from build123d import *

# Parameters (mm, degrees)
BOSS_EXTRUDE1_DEPTH      = 1.5875
BOSS_EXTRUDE1_DEPTH_BACK = 1.5875
SKETCH3_W                = 0.25
SKETCH3_H                = 13.334960838
SKETCH3_H_2              = 13.334960839
CUT_EXTRUDE1_DEPTH       = 103.531394128
SKETCH4_W                = 0.25
SKETCH4_H                = 6.667480419
SKETCH4_H_2              = 13.334960838
BOSS_EXTRUDE2_DEPTH      = 3.175


with BuildPart() as part:
    # Sketch2 → Boss-Extrude1 (new, two sides: drawn at the far end of the back side and taken through both)
    with BuildSketch(Plane(origin=(0, -26.564964534, 0), x_dir=(1, 0, 0), z_dir=(0, 1, 0)).offset(-BOSS_EXTRUDE1_DEPTH_BACK)):
        Polygon((-40, -26.352441257), (-40, -39.687402095), (-43.675, -39.687402095), (-43.675, -53.022362934), (-40, -53.022362934), (-40, -66.357323772), (-43.675, -66.357323772), (-43.675, -79.69228461), (-40, -79.69228461), (-40, -86.359765029), (-33.083333333, -86.359765029), (-33.083333333, -92.709765029), (-20.25, -92.709765029), (-20.25, -86.359765029), (-6.416666667, -86.359765029), (-6.416666667, -92.709765029), (6.416666667, -92.709765029), (6.416666667, -86.359765029), (20.25, -86.359765029), (20.25, -92.709765029), (33.083333333, -92.709765029), (33.083333333, -86.359765029), (40, -86.359765029), (40, -79.69228461), (43.675, -79.69228461), (43.675, -66.357323772), (40, -66.357323772), (40, -53.022362934), (43.675, -53.022362934), (43.675, -39.687402095), (40, -39.687402095), (40, -26.352441257), (43.675, -26.352441257), (43.675, -13.017480419), (40, -13.017480419), (40, -6.35), (33.083333333, -6.35), (33.083333333, 0), (20.25, 0), (20.25, -6.35), (6.416666667, -6.35), (6.416666667, 0), (-6.416666667, 0), (-6.416666667, -6.35), (-20.25, -6.35), (-20.25, 0), (-33.083333333, 0), (-33.083333333, -6.35), (-40, -6.35), (-40, -13.017480419), (-43.675, -13.017480419), (-43.675, -26.352441257), align=None)
    extrude(amount=BOSS_EXTRUDE1_DEPTH + BOSS_EXTRUDE1_DEPTH_BACK)

    # Sketch3 → Cut-Extrude1 (cut, through all)
    with BuildSketch(Plane(origin=(0, -24.977464534, 0), x_dir=(1, 0, 0), z_dir=(0, 1, 0))):
        with Locations((-43.55, -19.684960838)):
            Rectangle(SKETCH3_W, SKETCH3_H)
        with Locations((-43.55, -46.354882515)):
            Rectangle(SKETCH3_W, SKETCH3_H_2)
        with Locations((-43.55, -73.024804191)):
            Rectangle(SKETCH3_W, SKETCH3_H)
        with Locations((43.55, -19.684960838)):
            Rectangle(SKETCH3_W, SKETCH3_H)
        with Locations((43.55, -46.354882515)):
            Rectangle(SKETCH3_W, SKETCH3_H_2)
        with Locations((43.55, -73.024804191)):
            Rectangle(SKETCH3_W, SKETCH3_H)
    extrude(amount=-CUT_EXTRUDE1_DEPTH, mode=Mode.SUBTRACT)

    # Sketch4 → Boss-Extrude2 (add)
    with BuildSketch(Plane(origin=(0, -24.977464534, 0), x_dir=(1, 0, 0), z_dir=(0, 1, 0))):
        with Locations((-40.125, -9.683740209)):
            Rectangle(SKETCH4_W, SKETCH4_H)
        with Locations((-40.125, -33.019921676)):
            Rectangle(SKETCH4_W, SKETCH4_H_2)
        with Locations((-40.125, -59.689843353)):
            Rectangle(SKETCH4_W, SKETCH4_H_2)
        with Locations((-40.125, -83.02602482)):
            Rectangle(SKETCH4_W, SKETCH4_H)
        with Locations((40.125, -83.02602482)):
            Rectangle(SKETCH4_W, SKETCH4_H)
        with Locations((40.125, -59.689843353)):
            Rectangle(SKETCH4_W, SKETCH4_H_2)
        with Locations((40.125, -33.019921676)):
            Rectangle(SKETCH4_W, SKETCH4_H_2)
        with Locations((40.125, -9.683740209)):
            Rectangle(SKETCH4_W, SKETCH4_H)
    extrude(amount=-BOSS_EXTRUDE2_DEPTH)


solid = part.part
Verification items for the finished model (mm, model axes). A direction names the side the tool comes from. Coordinates: 2 decimals unless noted, no trailing zeros. Loops run counter-clockwise (first coordinate to the right, second up) from the corner with the lowest first, then second, coordinate; pieces in that order, holes last. Notation, with made-up numbers: (-35, -34.5) -> (18, -34.5) arc R27 cw to (18, 1.5) -> close; hole circle Ø1 at (62.5, 43.25). An arc over 180 degrees is marked (long way). Answer as a JSON object with one key per item and string values. Group by question number.
Item 1: Scan lines: probe 1 along X at (y, z) = (-27.8, 87); probe 2 along Z at (x, y) = (-13.5, -25.25); probe 3 along X at (y, z) = (-25.55, 10). Record each from-to range of solid material in increasing order.
Item 2: Tool access check on faces 1 (the flat face through (-13, -27, 86.36)), 2 (the flat face through (-40.25, -27, 83)), 3 (the flat face through (-40.25, -27, 60)), 4 (the flat face through (33.083, -27, 3)), 5 (the flat face through (6.417, -27, 3)). Record the directions out of +Z, -Z, +X, -X, +Y, -Y that give a thin tool (end or side, any length) a straight path to the whole face; none if there is none.
Item 3: Sectioned sample at A-A on x = -18. Record the boundary of the cut face in (y, z).
Item 4: Mould release check, pull along Z, two halves, no side actions. Record for faces 6 (the flat face through (0, -27, 92.71)), 7 (the flat face through (43.425, -27, 46)), 8 (the flat face through (-42, -27, 66.357)), 9 (the flat face through (-42, -27, 13.017)): +Z half, -Z half, draft (parallel to the pull), parting line (faces both ways), or undercut.
Item 5: Sectioned sample at B-B on z = 59. Record the boundary of the cut face in (x, y).
Item 6: Depth check by flat-ended pin: pin 1 (1 mm diameter, centred on x = -42, y = -27, fed in from +Z); pin 2 (1.6 mm diameter, centred on y = -26, z = 90, fed in from -X); pin 3 (1.6 mm diameter, centred on x = 42.5, y = -26, fed in from -Z). Enter the tip coordinate at first touch or a pass-through.
Evaluation:
{
 "1": {"probe 1": "x = -33.08 to -20.25, -6.42 to 6.42, 20.25 to 33.08", "probe 2": "z = 6.35 to 86.36", "probe 3": "x = -40.25 to 40.25"},
 "2": {"face 1": "+Z, +Y, -Y", "face 2": "+Z, -X, +Y, -Y", "face 3": "-X, +Y, -Y", "face 4": "-Z, +X, +Y, -Y", "face 5": "-Z, +Y, -Y"},
 "3": {"outline": "(-28.15, 6.35) -> (-24.98, 6.35) -> (-24.98, 86.36) -> (-28.15, 86.36) -> close"},
 "4": {"face 6": "+Z half", "face 7": "draft", "face 8": "undercut", "face 9": "-Z half"},
 "5": {"outline": "(-40.25, -28.15) -> (40.25, -28.15) -> (40.25, -24.98) -> (-40.25, -24.98) -> close"},
 "6": {"pin 1": "stops at z = 79.69", "pin 2": "stops at x = -33.08", "pin 3": "stops at z = 13.02"}
}
